Design review of the part built by this model. Coordinates are the model's own, in mm. A direction names the side the tool comes from. Coordinates: 2 decimals unless noted, no trailing zeros. Write each loop counter-clockwise with the first axis right and the second up, starting at its lowest first coordinate (ties: lowest second). Pieces come first, ordered by that corner, then holes. Notation, with made-up numbers: (30.25, 66) -> (35.25, 66) arc R34 cw to (35.25, 97) -> close; hole circle Ø2 at (52, -10.75). An arc over 180 degrees is marked (long way). Answer in a Markdown table with one row per item. Add a question column.
Item 1: For faces 1 (the face through (-1, 6.35, 2)), 2 (the face through (-2.901, 9.045, 1.683)), list the 3-axis set-ups (+Z, -Z, +X, -X, +Y, -Y) from which the entire face can be reached by the end or side of a thin tool; tool diameter is ignored.
Item 2: Take a section at A-A, the plane z = 0. Write out the cut boundary in (x, y) (3 decimals).
Item 3: To check wall thickness, follow line 1 (Y direction, x = -0.5, z = 2.5); line 2 (Z direction, x = 0, y = 4); line 3 (Z direction, x = -1.75, y = 3). State the ranges of each line that lie inside material, in increasing order.
Item 4: Take a section at B-B, the plane y = 5. Write out the cut boundary in (x, z).
Autodesk Inventor part; units mm, degrees
ref_plane "YZ Plane" through (0, 0, 0) normal (1, 0, 0) x (0, 1, 0)
ref_plane "XZ Plane" through (0, 0, 0) normal (0, 1, 0) x (-1, 0, 0)
ref_plane "XY Plane" through (0, 0, 0) normal (0, 0, 1) x (1, 0, 0)
sketch "Sketch1" plane through (0, 0, 0) normal (0, 1, 0) x (-1, 0, 0)
  circle A0 centre (0, 0) radius 2.0828
  dimension "d0" = 4.1656
extrude "Body" add sketch "Sketch1" along normal blind 6.35
sketch "Sketch2" plane through (0, 6.35, 0) normal (0, 1, 0) x (1, 0, 0)
  line L0 (-3.175, 1.8331) -> (0, 3.6662)
  line L1 (0, 3.6662) -> (3.175, 1.8331)
  line L2 (3.175, 1.8331) -> (3.175, -1.8331)
  line L3 (3.175, -1.8331) -> (0, -3.6662)
  line L4 (0, -3.6662) -> (-3.175, -1.8331)
  line L5 (-3.175, -1.8331) -> (-3.175, 1.8331)
  point P0 (0, 0)
  point P1 (0, 0)
  dimension "d3" = 6.35
extrude "Head" add sketch "Sketch2" along normal blind 2.794
sketch "Sketch3" plane through (0, 0, 0) normal (1, 0, 0) x (0, 1, 0)
  line L0 (8.8646, -3.6662) -> (9.144, -3.1822)
  line L1 (9.144, -3.1822) -> (9.144, -3.6662)
  line L2 (9.144, -3.6662) -> (8.8646, -3.6662)
  line L3 (6.35, -3.6662) -> (9.144, -3.6662)
  line L4 (9.144, -1.8331) -> (9.144, -3.6662)
  line L5 (-1.8288, 0) -> (10.9728, 0)
  point P0 (0, 0)
  dimension "d6" = 0.5588
  dimension "d7" = 60
revolve "Head Chamfer" cut sketch "Sketch3" angle 360 about axis through (0, -10, 0) along (0, 1, 0)
sketch "Sketch4" plane through (0, 0, 0) normal (0, 0, 1) x (1, 0, 0)
  line L0 (-2.0828, 0) -> (-2.0828, 6.35)
  line L1 (-2.0828, 0.0762) -> (-2.0828, -0.6413)
  line L2 (-2.0828, -0.6413) -> (-2.6162, -0.3334)
  line L3 (-2.6162, -0.3334) -> (-2.6162, -0.2318)
  line L4 (-2.6162, -0.2318) -> (-2.0828, 0.0762)
  line L5 (2.0828, 0) -> (-2.0828, 0)
  point P0 (0, 0)
  dimension "d9" = 60
  dimension "d10" = 0.1016
  dimension "d11" = 0.0762
  dimension "d12" = 0.5334
feature "Thread" [suppressed]
sketch "Sketch5" plane through (0, 0, 0) normal (0, 0, 1) x (1, 0, 0)
  line L0 (0, 0) -> (-1.4986, 0)
  line L1 (-1.4986, 0) -> (-2.2461, 0.7475)
  line L2 (-2.2461, 0.7475) -> (-2.2461, -1.8711)
  line L3 (-2.2461, -1.8711) -> (-1.4986, -1.8711)
  line L4 (-1.4986, -1.8711) -> (-1.4986, 0)
  line L5 (-2.0828, 0) -> (-2.0828, 0)
  line L6 (0, -2.3949) -> (0, 1.2713)
  point P0 (0, 0)
  dimension "d21" = 1.4986
  dimension "d22" = 135
  dimension "d23" = 0
  dimension "d24" = 0
revolve "Tapered End" cut sketch "Sketch5" angle 360 about axis through (0, -10, 0) along (0, 1, 0)
properties part number "Screw Nylon Hex" material "Black"
Answers:
| question | item | result |
|---|---|---|
| 1 | face 1 | -Y |
| 1 | face 2 | +Z, -X, +Y |
| 2 | outline | (-3.175, 6.35) -> (-2.083, 6.35) -> (-2.083, 0.584) -> (-1.499, 0) -> (1.499, 0) -> (2.083, 0.584) -> (2.083, 6.35) -> (3.175, 6.35) -> (3.175, 9.144) -> (-3.175, 9.144) -> close |
| 3 | line 1 | y = 6.35 to 9.14 |
| 3 | line 2 | z = -2.08 to 2.08 |
| 3 | line 3 | z = -1.13 to 1.13 |
| 4 | outline | circle Ø4.17 at (0, 0) |
